The figure shows three views and two pictorial views of one solid part (mm, origin at its lowest corner). Answer the questions. Round coordinates to 2 decimals unless told otherwise and drop trailing zeros. Loops run counter-clockwise (first coordinate to the right, second up) from the corner with the lowest first, then second, coordinate; pieces in that order, holes last. Notation, with made-up numbers: (58, 72) -> (65, 72) arc R36 cw to (65, 106) -> close; hole circle Ø1 at (12.25, 88.25). An arc over 180 degrees is marked (long way). Write item = value, one per line. Start each with the question number.
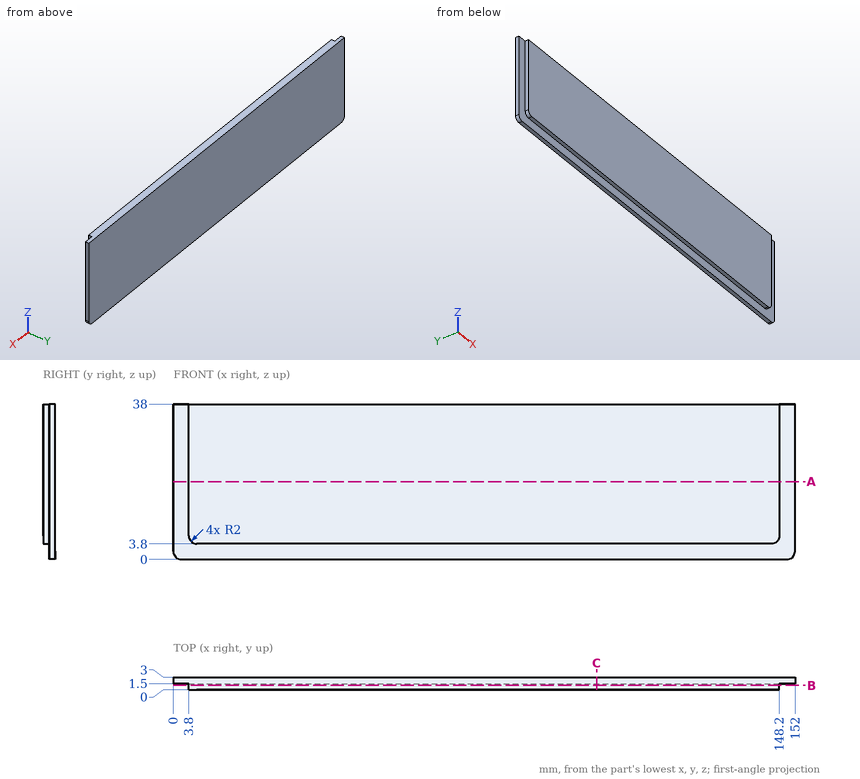
Item 1: Section C-C (x = 103.5) is taken. Determine the outline of the cut face in (y, z), then the cut area to 3 significant figures.
Item 2: Find the intervals of material crossed by line 1 along X through (y, z) = (0.5, 9); line 2 along Z through (x, y) = (75, 1.4); line 3 along X through (y, z) = (1.1, 4), in increasing order. Write a range as [from, to].
Item 3: Flat-ended cylindrical pins translate along their axes: pin 1 (0.8 mm diameter, centred on x = 77, y = 1, fed in from -Z); pin 2 (1.6 mm diameter, centred on y = 0.5, z = 29.5, fed in from +X); pin 3 (0.8 mm diameter, centred on y = 0.5, z = 17.5, fed in from -X). Find the tip coordinate at first contact, or state that the pin passes through.
Item 4: Section B-B (y = 1.05) is taken. Determine the outline of the cut face in (x, z), then the cut area to 3 significant figures.
Item 5: Section A-A (z = 19) is taken. Determine the outline of the cut face in (x, y), then the cut area to 3 significant figures.
Worked answers:
q1.outline = (0, 3.8) -> (1.5, 3.8) -> (1.5, 0) -> (3, 0) -> (3, 38) -> (0, 38) -> close
q1.area = 108 mm2
q2.line_1 = [3.8, 148.2]
q2.line_2 = [3.8, 38]
q2.line_3 = [4.93, 147.07]
q3.pin_1 = 3.8
q3.pin_2 = 148.2
q3.pin_3 = 3.8
q4.outline = (3.8, 5.8) arc R2 ccw to (5.8, 3.8) -> (146.2, 3.8) arc R2 ccw to (148.2, 5.8) -> (148.2, 38) -> (3.8, 38) -> close
q4.area = 4,940 mm2
q5.outline = (0, 1.5) -> (3.8, 1.5) -> (3.8, 0) -> (148.2, 0) -> (148.2, 1.5) -> (152, 1.5) -> (152, 3) -> (0, 3) -> close
q5.area = 445 mm2
